```python
from build123d import *

# Parameters (mm, degrees)
SKETCH1_R           = 0.5
BOSS_EXTRUDE1_DEPTH = 0.19


with BuildPart() as part:
    # Sketch1 → Boss-Extrude1 (new body)
    with BuildSketch(Plane(origin=(0, 0, 0), x_dir=(1, 0, 0), z_dir=(0, 1, 0))):
        with BuildLine():
            Line((70.757013136, 151.738904346), (70.334205326, 150.83219007))
            ThreePointArc((70.334205326, 150.83219007), (70.142130859, 147.07974632), (72.617523713, 144.253059759))
            ThreePointArc((72.617523713, 144.253059759), (114.197745162, 114.197745162), (144.253059759, 72.617523713))
            ThreePointArc((144.253059759, 72.617523713), (147.07974632, 70.142130859), (150.83219007, 70.334205326))
            Line((150.83219007, 70.334205326), (151.738904346, 70.757013136))
            ThreePointArc((151.738904346, 70.757013136), (155.63203997, 70.897887093), (158.44459254, 68.202354028))
            ThreePointArc((158.44459254, 68.202354028), (172.5, 0), (158.44459254, -68.202354028))
            ThreePointArc((158.44459254, -68.202354028), (155.63203997, -70.897887093), (151.738904346, -70.757013136))
            Line((151.738904346, -70.757013136), (150.83219007, -70.334205326))
            ThreePointArc((150.83219007, -70.334205326), (147.07974632, -70.142130859), (144.253059759, -72.617523713))
            ThreePointArc((144.253059759, -72.617523713), (114.197745162, -114.197745162), (72.617523713, -144.253059759))
            ThreePointArc((72.617523713, -144.253059759), (70.142130859, -147.07974632), (70.334205326, -150.83219007))
            Line((70.334205326, -150.83219007), (70.757013136, -151.738904346))
            ThreePointArc((70.757013136, -151.738904346), (70.897887093, -155.63203997), (68.202354028, -158.44459254))
            ThreePointArc((68.202354028, -158.44459254), (0, -172.5), (-68.202354028, -158.44459254))
            ThreePointArc((-68.202354028, -158.44459254), (-70.897887093, -155.63203997), (-70.757013136, -151.738904346))
            Line((-70.757013136, -151.738904346), (-70.334205326, -150.83219007))
            ThreePointArc((-70.334205326, -150.83219007), (-70.142130859, -147.07974632), (-72.617523713, -144.253059759))
            ThreePointArc((-72.617523713, -144.253059759), (-114.197745162, -114.197745162), (-144.253059759, -72.617523713))
            ThreePointArc((-144.253059759, -72.617523713), (-147.07974632, -70.142130859), (-150.83219007, -70.334205326))
            Line((-150.83219007, -70.334205326), (-151.738904346, -70.757013136))
            ThreePointArc((-151.738904346, -70.757013136), (-155.63203997, -70.897887093), (-158.44459254, -68.202354028))
            ThreePointArc((-158.44459254, -68.202354028), (-172.5, 0), (-158.44459254, 68.202354028))
            ThreePointArc((-158.44459254, 68.202354028), (-155.63203997, 70.897887093), (-151.738904346, 70.757013136))
            Line((-151.738904346, 70.757013136), (-150.83219007, 70.334205326))
            ThreePointArc((-150.83219007, 70.334205326), (-147.07974632, 70.142130859), (-144.253059759, 72.617523713))
            ThreePointArc((-144.253059759, 72.617523713), (-114.197745162, 114.197745162), (-72.617523713, 144.253059759))
            ThreePointArc((-72.617523713, 144.253059759), (-70.142130859, 147.07974632), (-70.334205326, 150.83219007))
            Line((-70.334205326, 150.83219007), (-70.757013136, 151.738904346))
            ThreePointArc((-70.757013136, 151.738904346), (-70.897887093, 155.63203997), (-68.202354028, 158.44459254))
            ThreePointArc((-68.202354028, 158.44459254), (0, 172.5), (68.202354028, 158.44459254))
            ThreePointArc((68.202354028, 158.44459254), (70.897887093, 155.63203997), (70.757013136, 151.738904346))
        make_face()
        with Locations(Location((-64.290816637, 155.211761462, 0), (0, 0, 270))):
            Circle(SKETCH1_R, mode=Mode.SUBTRACT)
        with Locations(Location((64.290816637, 155.211761462, 0), (0, 0, 270))):
            Circle(SKETCH1_R, mode=Mode.SUBTRACT)
        with Locations(Location((155.211761462, 64.290816637, 0), (0, 0, 270))):
            Circle(SKETCH1_R, mode=Mode.SUBTRACT)
        with Locations(Location((155.211761462, -64.290816637, 0), (0, 0, 270))):
            Circle(SKETCH1_R, mode=Mode.SUBTRACT)
        with Locations(Location((64.290816637, -155.211761462, 0), (0, 0, 270))):
            Circle(SKETCH1_R, mode=Mode.SUBTRACT)
        with Locations(Location((-64.290816637, -155.211761462, 0), (0, 0, 270))):
            Circle(SKETCH1_R, mode=Mode.SUBTRACT)
        with Locations(Location((-155.211761462, -64.290816637, 0), (0, 0, 270))):
            Circle(SKETCH1_R, mode=Mode.SUBTRACT)
        with Locations(Location((-155.211761462, 64.290816637, 0), (0, 0, 270))):
            Circle(SKETCH1_R, mode=Mode.SUBTRACT)
    extrude(amount=BOSS_EXTRUDE1_DEPTH)


solid = part.part
```
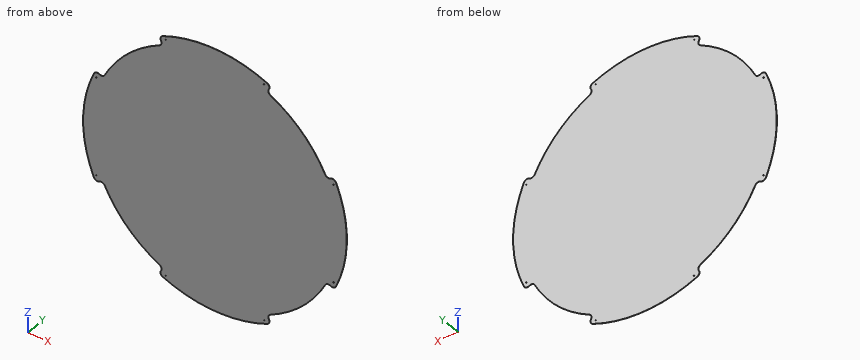
Here's how the part is built. I have some questions about the finished solid (model axes, mm). Round coordinates to 2 decimals unless told otherwise and drop trailing zeros. Loops run counter-clockwise (first coordinate to the right, second up) from the corner with the lowest first, then second, coordinate; pieces in that order, holes last.
1. If I drill on probe 1 along X at (y, z) = (0.05, -48); probe 2 along Z at (x, y) = (-20, 0.1); probe 3 along X at (y, z) = (0.1, 134), over which ranges is the centre line in solid material (lowest first)?
Answers:
probe 1: x = -165.69 to 165.69
probe 2: z = -171.34 to 171.34
probe 3: x = -90.15 to 90.15
2. Suppose I cut it at C-C, the plane y = 0.15. Give the number of separate pieces and of enclosed holes in the cut face, and give its area (3 significant figures).
Answers:
separate pieces: 1
enclosed holes: 8
area: 88,300 mm2
3. Suppose I cut it at B-B, the plane x = 98. Please give me the cut outline in (y, z).
Answers:
outline: (0, -128.37) - (0.19, -128.37) - (0.19, 128.37) - (0, 128.37) - close
4. Suppose I cut it at A-A, the plane z = 83.5. Please give me the cut outline in (x, y), and give its area (3 significant figures).
Answers:
outline: (-138.24, 0) - (138.24, 0) - (138.24, 0.19) - (-138.24, 0.19) - close
area: 52.5 mm2
